```python
from build123d import *

# Parameters (mm, degrees)
BOSS_EXTRUDE2_DEPTH = 5
CUT_EXTRUDE1_REACH  = 176.937
SKETCH2_R           = 2.2


with BuildPart() as part:
    # Sketch1 → Boss-Extrude2 (new body)
    with BuildSketch(Plane(origin=(0, 0, 0), x_dir=(1, 0, 0), z_dir=(0, 1, 0))):
        with BuildLine():
            ThreePointArc((-26.256294904, 162.782156045), (-34.757388509, 167.168565439), (-41.482617684, 160.365590178))
            Line((-41.482617684, 160.365590178), (-50.932711484, 96.056215067))
            ThreePointArc((-50.932711484, 96.056215067), (-50.956557115, 95.796817406), (-50.979081843, 95.537301709))
            add(Edge.make_bspline(
                [(-22.456551163, 100.599709115), (-25.176477923, 89.862155319), (-41.371339617, 77.714728994), (-51.090796969, 92.352457993), (-50.979081843, 95.537301709)],
                knots=[0, 0, 0, 0, 0.694817922, 0.98396673, 0.98396673, 0.98396673, 0.98396673], degree=3))
            ThreePointArc((-22.456551163, 100.599709115), (-18.824269383, 120.221092129), (-17.76802696, 140.147870449))
            ThreePointArc((-17.76802696, 140.147870449), (-17.943181625, 142.067888002), (-18.417828761, 143.936539027))
            ThreePointArc((-18.417828761, 143.936539027), (-22.023480215, 153.489775682), (-26.256294904, 162.782156045))
        make_face()
    extrude(amount=BOSS_EXTRUDE2_DEPTH)

    # Sketch2 → Cut-Extrude1 (cut, up to next)
    with BuildSketch(Plane(origin=(0, 5, 0), x_dir=(1, 0, 0), z_dir=(0, 1, 0)), mode=Mode.PRIVATE) as cut_extrude1_sk1:
        with Locations(Location((-31, 140, 0), (0, 0, 270))):
            Circle(SKETCH2_R)
    cut_extrude1_tool1 = extrude(cut_extrude1_sk1.sketch, amount=-CUT_EXTRUDE1_REACH, mode=Mode.PRIVATE) & part.part
    # Sketch2 → Cut-Extrude1 (cut, up to next)
    with BuildSketch(Plane(origin=(0, 5, 0), x_dir=(1, 0, 0), z_dir=(0, 1, 0)), mode=Mode.PRIVATE) as cut_extrude1_sk2:
        with Locations(Location((-38, 110, 0), (0, 0, 270))):
            Circle(SKETCH2_R)
    cut_extrude1_tool2 = extrude(cut_extrude1_sk2.sketch, amount=-CUT_EXTRUDE1_REACH, mode=Mode.PRIVATE) & part.part
    add(cut_extrude1_tool1.solids().sort_by_distance((-31, 5, -140))[0], mode=Mode.SUBTRACT)
    add(cut_extrude1_tool2.solids().sort_by_distance((-38, 5, -110))[0], mode=Mode.SUBTRACT)


solid = part.part
```
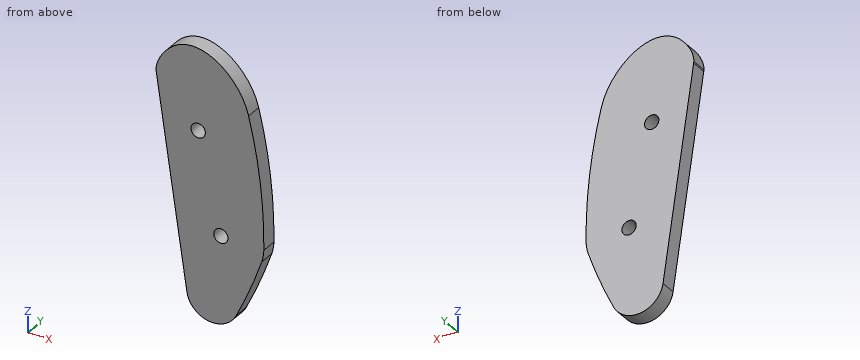
Here's how the part is built. I have some questions about the finished solid (model axes, mm). Coordinates: 2 decimals unless noted, no trailing zeros. Order: outer loops, then holes, each group sorted by start corner. A loop starts at its lowest first (then second) coordinate and runs counter-clockwise, first axis right, second up. Notation, with made-up numbers: (10, 15) -> (54, 15) arc R18 ccw to (54, 27) -> close; hole circle Ø9 at (65, 35.5). An arc over 180 degrees is marked (long way). Return JSON: item names as keys, results as strings.
1) If we section it at B-B on y = 0.8: State how many separate pieces and enclosed holes the cut face has, plus the area to 3 significant figures.
Conclusion:
{"separate pieces": "1", "enclosed holes": "2", "area": "1,960 mm²"}
2) If I drill on probe 1 along Z at (x, y) = (-36, 2.8); probe 2 along X at (y, z) = (1.05, -140); probe 3 along Z at (x, y) = (-33, 4.5), over which ranges is the centre line in solid material (lowest first)?
Conclusion:
{"probe 1": "z = -166.87 to -110.92, -109.08 to -85.31", "probe 2": "x = -44.48 to -33.2, -28.8 to -17.77", "probe 3": "z = -167.25 to -140.92, -139.08 to -86.63"}
3) If we section it at C-C on x = -20.5: List the corners of the cut face in (y, z) for me.
Conclusion:
{"outline": "(0, -149.68) -> (5, -149.68) -> (5, -109.4) -> (0, -109.4) -> close"}
4) I'm going to push flat-ended pins straight in: P1, Ø2.5, axis at x = -38, z = -110, coming from the +Y side; P2, Ø1, axis at x = -31.5, y = 1.5, coming from the -Z side; P3, Ø1.5, axis at y = 2.5, z = -93, coming from the -X side. Where does each tip first touch, or does it pass through?
Conclusion:
{"P1": "passes through", "P2": "stops at z = -167.13", "P3": "stops at x = -50.77"}
5) If we section it at D-D on z = -118.5: List the corners of the cut face in (x, y) for me.
Conclusion:
{"outline": "(-47.63, 0) -> (-19.04, 0) -> (-19.04, 5) -> (-47.63, 5) -> close"}
6) If we section it at A-A on z = -109.5: List the corners of the cut face in (x, y) for me, plus the area to 3 significant figures.
Conclusion:
{"outline": "(-48.96, 0) -> (-40.14, 0) -> (-40.14, 5) -> (-48.96, 5) -> close; (-35.86, 0) -> (-20.48, 0) -> (-20.48, 5) -> (-35.86, 5) -> close", "area": "121 mm²"}
